from build123d import *

# Parameters (mm, degrees)
SKETCH1_W           = 20
SKETCH1_H           = 28
BOSS_EXTRUDE1_DEPTH = 1
FILLET1_R           = 2
SKETCH2_W           = 25.473591578
SKETCH2_H           = 30.562755328
CUT_EXTRUDE1_DEPTH  = 18.23368794
SKETCH3_R           = 1.6
CUT_EXTRUDE2_DEPTH  = 18.094443542
CUT_EXTRUDE3_DEPTH  = 10


with BuildPart() as part:
    # Sketch1 → Boss-Extrude1 (new body)
    with BuildSketch(Plane(origin=(0, 0, 0), x_dir=(1, 0, 0), z_dir=(0, 1, 0))):
        Rectangle(SKETCH1_W, SKETCH1_H)
    extrude(amount=BOSS_EXTRUDE1_DEPTH)

    # Fillet1
    fillet1_edges = [part.edges().sort_by_distance(p)[0] for p in [
        (10, 0.5, 14),
        (-10, 0.5, 14),
        (-10, 0.5, -14),
        (10, 0.5, -14),
    ]]
    fillet(fillet1_edges, radius=FILLET1_R)

    # Sketch2 → Cut-Extrude1 (cut, through all)
    with BuildSketch(Plane(origin=(0, 1, 0), x_dir=(1, 0, 0), z_dir=(0, 1, 0))):
        Rectangle(SKETCH2_W, SKETCH2_H)
        with BuildLine():
            Line((-8, -13.9), (8, -13.9))
            ThreePointArc((8, -13.9), (9.343502884, -13.343502884), (9.9, -12))
            Line((9.9, -12), (9.9, 12))
            ThreePointArc((9.9, 12), (9.343502884, 13.343502884), (8, 13.9))
            Line((8, 13.9), (-8, 13.9))
            ThreePointArc((-8, 13.9), (-9.343502884, 13.343502884), (-9.9, 12))
            Line((-9.9, 12), (-9.9, -12))
            ThreePointArc((-9.9, -12), (-9.343502884, -13.343502884), (-8, -13.9))
        make_face(mode=Mode.SUBTRACT)
    extrude(amount=-CUT_EXTRUDE1_DEPTH, mode=Mode.SUBTRACT)

    # Sketch3 → Cut-Extrude2 (cut, through all)
    with BuildSketch(Plane(origin=(0, 0, 0), x_dir=(-1, 0, 0), z_dir=(0, -1, 0))):
        with Locations(Location((6, -10.5, 0), (0, 0, 90))):
            Circle(SKETCH3_R)
        with Locations(Location((6, 10.5, 0), (0, 0, 90))):
            Circle(SKETCH3_R)
    extrude(amount=-CUT_EXTRUDE2_DEPTH, mode=Mode.SUBTRACT)

    # Sketch4 → Cut-Extrude3 (cut)
    with BuildSketch(Plane(origin=(0, 1, 0), x_dir=(1, 0, 0), z_dir=(0, 1, 0))):
        with BuildLine():
            Line((2.5, 6), (2.5, -6))
            ThreePointArc((2.5, -6), (0, -8.5), (-2.5, -6))
            Line((-2.5, -6), (-2.5, 6))
            ThreePointArc((-2.5, 6), (0, 8.5), (2.5, 6))
        make_face()
    extrude(amount=-CUT_EXTRUDE3_DEPTH, mode=Mode.SUBTRACT)


solid = part.part
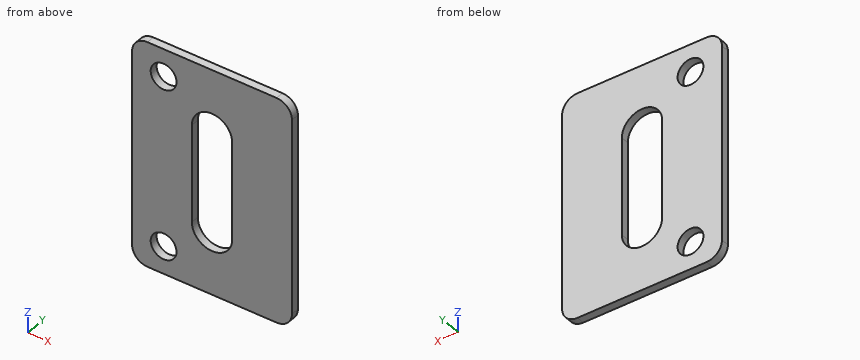
The listing builds one solid part. Answer for the finished solid, in the listing's coordinates (mm). Coordinates: 2 decimals unless noted, no trailing zeros. Loops run counter-clockwise (first coordinate to the right, second up) from the corner with the lowest first, then second, coordinate; pieces in that order, holes last. Notation, with made-up numbers: (60.25, 5) -> (85.25, 5) arc R15 cw to (85.25, 13) -> close; hole circle Ø3 at (53, -28). An arc over 180 degrees is marked (long way). Write item = value, one per line. Start each with the question number.
1) A cutting plane is placed at C-C (z = -5). Give the vertices of the cut face in (x, y).
2) Given pin 1 Ø1.9 at (x, z) = (-6, 10.5) entering from +Y, flat-ended and moving along its own axis, determine where the tip first touches the part or whether it passes through.
3) A cutting plane is placed at A-A (x = 0). Give the vertices of the cut face in (y, z), then the cut area to 3 significant figures.
4) A cutting plane is placed at B-B (y = 0.4). Give the vertices of the cut face in (x, z).
5) Straight lines are drawn through the part: line 1 (X direction, y = 0.35, z = -10.5); line 2 (X direction, y = 0.2, z = -5.5); line 3 (Z direction, x = -5.5, y = 0.85). For each, find the intervals that lie inside material, in ascending order. Write a range as from..to.
Responses:
q1.outline = (-9.9, 0) -> (-2.5, 0) -> (-2.5, 1) -> (-9.9, 1) -> close; (2.5, 0) -> (9.9, 0) -> (9.9, 1) -> (2.5, 1) -> close
q2.pin_1 = through
q3.outline = (0, -13.9) -> (1, -13.9) -> (1, -8.5) -> (0, -8.5) -> close; (0, 8.5) -> (1, 8.5) -> (1, 13.9) -> (0, 13.9) -> close
q3.area = 10.8 mm²
q4.outline = (-9.9, -12) arc R1.9 ccw to (-8, -13.9) -> (8, -13.9) arc R1.9 ccw to (9.9, -12) -> (9.9, 12) arc R1.9 ccw to (8, 13.9) -> (-8, 13.9) arc R1.9 ccw to (-9.9, 12) -> close; hole circle Ø3.2 at (-6, -10.5); hole circle Ø3.2 at (-6, 10.5); hole (-2.5, -6) arc R2.5 ccw to (2.5, -6) -> (2.5, 6) arc R2.5 ccw to (-2.5, 6) -> close
q5.line_1 = -9.9..-7.6, -4.4..9.9
q5.line_2 = -9.9..-2.5, 2.5..9.9
q5.line_3 = -13.9..-12.02, -8.98..8.98, 12.02..13.9
